Geometry check sheet. Reference: the model listing, model coordinates, mm. Face numbers are marked on the shaded views. A direction names the side the tool comes from. Round coordinates to 2 decimals unless told otherwise and drop trailing zeros. Order: outer loops, then holes, each group sorted by start corner. A loop starts at its lowest first (then second) coordinate and runs counter-clockwise, first axis right, second up. Notation, with made-up numbers: (-22, 84) - (1, 84) arc R16 ccw to (1, 99) - close; hole circle Ø9 at (59.25, 18). An arc over 180 degrees is marked (long way). One line per question, with ' | ' between items. Start each with the question number.
Q1. Material ranges on line 1 along X through (y, z) = (0.25, 16) (3 decimals); line 2 along Z through (x, y) = (-8, -3.5) (3 decimals), recorded low to high.
Q2. Sectioned sample at C-C, the plane x = -1.75. Enter the section's corners in (y, z) (3 decimals).
Q3. Mould release check, pull along X, two halves, no side actions. Record for the marked faces 1, 2, 3 and 4: +X half, -X half, draft (parallel to the pull), parting line (faces both ways), or undercut.
Q4. Sectioned sample at D-D, the plane z = 2.25. Enter the section's corners in (x, y) (3 decimals), then the cut area to 3 significant figures.
Q5. Tool access check on the marked faces 5, 6 and 7. Record the directions out of +Z, -Z, +X, -X, +Y, -Y that give a thin tool (end or side, any length) a straight path to the whole face; none if there is none.
Q6. Sectioned sample at B-B, the plane y = 5.5. Enter the section's corners in (x, z) (3 decimals), then the cut area to 3 significant figures.
Q7. Gauge pin test, flat ends, axial feed: P1, Ø1.8, axis at x = -3, y = 8.5, coming from the +Z side (3 decimals); P2, Ø3, axis at x = 5, y = -7.5, coming from the -Z side. Record the tip position at first contact, or that the pin passes through.
Q8. Sectioned sample at A-A, the plane y = 0. Enter the section's corners in (x, z) (1 decimal), then the cut area to 3 significant figures.
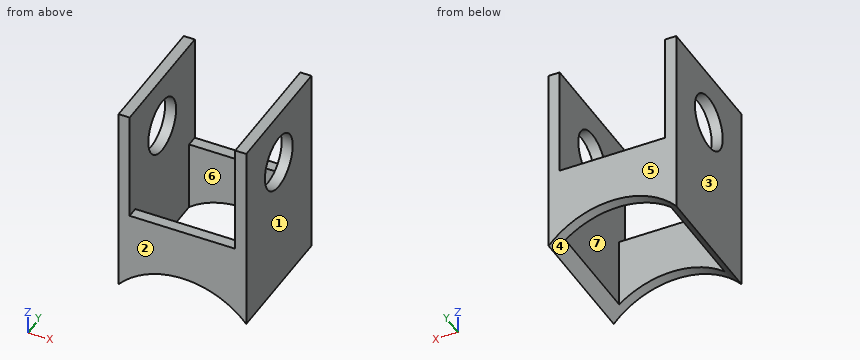
```python
from build123d import *

# Parameters (mm, degrees)
SKETCH1_W               = 19.05
SKETCH1_H               = 19.05
SKETCH1_W_2             = 15.748
SKETCH1_H_2             = 15.748
BOSS_EXTRUDE1_DEPTH     = 28.575
CUT_EXTRUDE5_DEPTH      = 36.639286609
CUT_EXTRUDE5_DEPTH_BACK = 36.639286609
SKETCH5_R               = 12.7
CUT_EXTRUDE2_DEPTH      = 36.639286609
CUT_EXTRUDE2_DEPTH_BACK = 36.639286609
SKETCH3_R               = 4.064
CUT_EXTRUDE4_DEPTH      = 36.639286609
CUT_EXTRUDE4_DEPTH_BACK = 36.639286609
SKETCH4_W               = 15.748
SKETCH4_H               = 16.51


with BuildPart() as part:
    # Sketch1 → Boss-Extrude1 (new body)
    with BuildSketch(Plane.XY):
        Rectangle(SKETCH1_W, SKETCH1_H)
        Rectangle(SKETCH1_W_2, SKETCH1_H_2, mode=Mode.SUBTRACT)
    extrude(amount=BOSS_EXTRUDE1_DEPTH)

    # Sketch5 → Cut-Extrude5 (cut, two sides: drawn at the far end of the back side and taken through both)
    with BuildSketch(Plane(origin=(0, 9.525, 0), x_dir=(1, 0, 0), z_dir=(0, 1, 0)).offset(-CUT_EXTRUDE5_DEPTH_BACK)):
        with Locations((0, 8.400260413)):
            Circle(SKETCH5_R)
    extrude(amount=CUT_EXTRUDE5_DEPTH + CUT_EXTRUDE5_DEPTH_BACK, mode=Mode.SUBTRACT)

    # Sketch3 → Cut-Extrude2 (cut, two sides: drawn at the far end of the back side and taken through both)
    with BuildSketch(Plane(origin=(9.525, 0, 0), x_dir=(0, 0, -1), z_dir=(1, 0, 0)).offset(-CUT_EXTRUDE2_DEPTH_BACK)):
        with Locations(Location((-20.6375, 0, 0), (0, 0, 90))):
            Circle(SKETCH3_R)
    extrude(amount=CUT_EXTRUDE2_DEPTH + CUT_EXTRUDE2_DEPTH_BACK, mode=Mode.SUBTRACT)

    # Sketch4 → Cut-Extrude4 (cut, two sides: drawn at the far end of the back side and taken through both)
    with BuildSketch(Plane.XZ.offset(9.525).offset(-CUT_EXTRUDE4_DEPTH_BACK)):
        with Locations((0, 20.32)):
            Rectangle(SKETCH4_W, SKETCH4_H)
    extrude(amount=CUT_EXTRUDE4_DEPTH + CUT_EXTRUDE4_DEPTH_BACK, mode=Mode.SUBTRACT)


solid = part.part
```
Determined:
1) line 1: x = -9.525 to -7.874, 7.874 to 9.525 | line 2: z = 1.463 to 18.572, 22.703 to 28.575
2) outline: (-9.525, 4.179) - (-7.874, 4.179) - (-7.874, 12.065) - (-9.525, 12.065) - close; (7.874, 4.179) - (9.525, 4.179) - (9.525, 12.065) - (7.874, 12.065) - close
3) face 1: +X half | face 2: draft | face 3: -X half | face 4: undercut
4) outline: (-9.525, -9.525) - (-6.918, -9.525) - (-6.918, -7.874) - (-7.874, -7.874) - (-7.874, 7.874) - (-6.918, 7.874) - (-6.918, 9.525) - (-9.525, 9.525) - close; (6.918, -9.525) - (9.525, -9.525) - (9.525, 9.525) - (6.918, 9.525) - (6.918, 7.874) - (7.874, 7.874) - (7.874, -7.874) - (6.918, -7.874) - close | area: 69.2 mm2
5) face 5: +Z, -Z, +X, -X, +Y | face 6: +Z, -Z | face 7: +Z
6) outline: (-9.525, 0) arc R12.7 cw to (-7.874, 1.564) - (-7.874, 28.575) - (-9.525, 28.575) - close; (7.874, 1.564) arc R12.7 cw to (9.525, 0) - (9.525, 28.575) - (7.874, 28.575) - close | area: 91.6 mm2
7) P1: stops at z = 12.065 | P2: stops at z = 2.54
8) outline: (-9.5, 0) arc R12.7 cw to (-7.9, 1.6) - (-7.9, 16.6) - (-9.5, 16.6) - close; (-9.5, 24.7) - (-7.9, 24.7) - (-7.9, 28.6) - (-9.5, 28.6) - close; (7.9, 1.6) arc R12.7 cw to (9.5, 0) - (9.5, 16.6) - (7.9, 16.6) - close; (7.9, 24.7) - (9.5, 24.7) - (9.5, 28.6) - (7.9, 28.6) - close | area: 64.8 mm2
